For this review, take the finished solid that the model builds, in its own axes (mm). A direction names the side the tool comes from. Round coordinates to 2 decimals unless told otherwise and drop trailing zeros. Loops run counter-clockwise (first coordinate to the right, second up) from the corner with the lowest first, then second, coordinate; pieces in that order, holes last. Notation, with made-up numbers: (50.25, 27.5) -> (80.25, 27.5) arc R23 ccw to (80.25, 36.5) -> close; hole circle Ø1 at (-3, 29.25). An arc over 180 degrees is marked (long way). Write each question's results on one line, items separated by ' | '.
Autodesk Inventor part; units mm, degrees
ref_plane "YZ Plane" through (0, 0, 0) normal (1, 0, 0) x (0, 1, 0)
ref_plane "XZ Plane" through (0, 0, 0) normal (0, 1, 0) x (-1, 0, 0)
ref_plane "XY Plane" through (0, 0, 0) normal (0, 0, 1) x (1, 0, 0)
sketch "스케치1" plane through (0, 0, 0) normal (0, 1, 0) x (-1, 0, 0)
  line L0 (270, 0) -> (-270, 0)
  line L1 (270, 0) -> (270, -240)
  line L2 (270, -240) -> (230, -240)
  line L3 (230, -240) -> (230, -40)
  line L4 (230, -40) -> (-230, -40)
  line L5 (-230, -40) -> (-230, -240)
  line L6 (-230, -240) -> (-270, -240)
  line L7 (-270, -240) -> (-270, 0)
  line L8 (-560, -240) -> (480, -240)
  arc A0 (360, -240) -> (520, -80) centre (360, -80) ccw
  arc A1 (360, -140) -> (420, -80) centre (360, -80) ccw
  line L9 (420, -80) -> (520, -80)
  line L10 (360, -140) -> (-40, -140)
  arc A2 (-520, -80) -> (-360, -240) centre (-360, -80) ccw
  arc A3 (-420, -80) -> (-360, -140) centre (-360, -80) ccw
  line L11 (-420, -80) -> (-520, -80)
  line L12 (-360, -140) -> (-40, -140)
  line L13 (360, -240) -> (-360, -240)
  point P0 (0, 0)
  point P1 (0, 0)
  point P2 (-270, -140)
  point P3 (-230, -140)
  point P4 (230, -140)
  point P5 (270, -140)
  dimension "d1" = 240
  dimension "d2" = 40
  dimension "d3" = 200
  dimension "d4" = 460
  dimension "d6" = 1040
  dimension "d9" = 240
  dimension "d11" = 100
  dimension "d12" = 160
  dimension "d13" = 160
  dimension "d14" = 160
  dimension "d17" = 210
  dimension "d18" = 310
  dimension "d24" = 270
  dimension "d25" = 0
  dimension "d26" = 250
  dimension "d27" = 60
  dimension "d28" = 0
  dimension "d29" = 160
  dimension "d30" = 0
  dimension "d31" = 60
  dimension "d32" = 40
  dimension "d33" = 160
  dimension "d34" = 40
  dimension "d35" = 60
  dimension "d36" = 500
  dimension "d37" = 160
  dimension "d38" = 500
  dimension "d39" = 60
  dimension "d40" = 540
  dimension "d41" = 160
  dimension "d42" = 540
  dimension "d43" = 630
  dimension "d44" = 160
  dimension "d45" = 630
extrude "돌출3" add sketch "스케치1" along normal mid plane 40 contours L1 L10 L3 L4 L5 L12 L7 L0
extrude "돌출4" add sketch "스케치1" along normal mid plane 100 contours L10 A1 L9 A0 L8 L1 | L1 L2 L3 L10 | L12 L5 L6 L7 | L7 L8 A2 L11 A3 L12 | L3 L8 L5 L12 L10
fillet "모깎기1" radius 20 18 edges at (-473.1371, 50, -193.1371) (473.1371, 50, -193.1371) (-473.1371, -50, -193.1371) (473.1371, -50, -193.1371) (470, 50, -80) (402.4264, 50, -122.4264) (-402.4264, 50, -122.4264) (0, 50, -140) (470, -50, -80) (-402.4264, -50, -122.4264) (402.4264, -50, -122.4264) (0, -50, -140) (-470, -50, -80) (-470, 50, -80) (-520, 0, -80) (-420, 0, -80) (420, 0, -80) (520, 0, -80)
properties part number "bumper"
1. For pin 1 (1.5 mm diameter, centred on x = -95.5, y = -33.5, fed in from +Z); pin 2 (6 mm diameter, centred on y = 16, z = -78.5, fed in from +X); pin 3 (6 mm diameter, centred on y = -31.5, z = -118.5, fed in from +X), all flat-tipped, find the tip position at first contact; note any pin that passes through.
Values found:
pin 1: stops at z = -140.19 | pin 2: stops at x = 506.16 | pin 3: stops at x = 515.98
2. Consider section B-B (y = 4.5). State the section outline as (x, z) points, plus the area to 3 significant figures.
Values found:
outline: (-518.36, -102.86) arc R160 ccw to (-360, -240) -> (360, -240) arc R160 ccw to (518.36, -102.86) arc R20 ccw to (498.56, -80) -> (437.46, -80) arc R20 ccw to (418.09, -95) arc R60 cw to (360, -140) -> (270, -140) -> (270, 0) -> (-270, 0) -> (-270, -140) -> (-360, -140) arc R60 cw to (-418.09, -95) arc R20 ccw to (-437.46, -80) -> (-498.56, -80) arc R20 ccw to start; hole (-230, -140) -> (230, -140) -> (230, -40) -> (-230, -40) -> close | area: 136,000 mm2
3. Draft analysis for pull direction Z (two halves, no side actions). For faces 1 (the face through (-468.44, 43.986, -85.703)), 2 (the face through (-3, 0, -40)), 3 (the face through (-465.948, -0.42, -199.896)), state which applies: released by +Z, released by -Z, zero draft, split by the parting line, or undercut.
Values found:
face 1: released by +Z | face 2: undercut | face 3: released by -Z
4. To check wall thickness, follow probe 1 along X at (y, z) = (-10.5, -42.5); probe 2 along Z at (x, y) = (-143, 13.5); probe 3 along Z at (x, y) = (-335.5, -29.5). State the ranges of each line that lie inside material, in increasing order.
Values found:
probe 1: x = -270 to -230, 230 to 270 | probe 2: z = -240 to -140, -40 to 0 | probe 3: z = -240 to -140
5. Consider section C-C (z = -19). State the section outline as (x, y) points.
Values found:
outline: (-270, -20) -> (270, -20) -> (270, 20) -> (-270, 20) -> close
6. Consider section A-A (x = 175.5). State the section outline as (y, z) points.
Values found:
outline: (-50, -220) arc R20 ccw to (-30, -240) -> (30, -240) arc R20 ccw to (50, -220) -> (50, -160) arc R20 ccw to (30, -140) -> (-30, -140) arc R20 ccw to (-50, -160) -> close; (-20, -40) -> (20, -40) -> (20, 0) -> (-20, 0) -> close
7. Tool access review of faces 4 (the face through (-270, 0, -69)), 5 (the face through (-5.04, -43.986, -234.297)), 6 (the face through (7, 50, -172)), 7 (the face through (468, 0, -80)), 8 (the face through (4, -20, -38)): name each direction out of +Z, -Z, +X, -X, +Y, -Y from which nothing blocks a thin tool from reaching the whole face with its end or side.
Values found:
face 4: +Z, +Y, -Y | face 5: -Z, +X, -X, -Y | face 6: +Z, -Z, +X, -X, +Y | face 7: +Z, +X, +Y, -Y | face 8: +Z, -Y
